For this review, take the finished solid that the model builds, in its own axes (mm). Face numbers are marked on the shaded views. A direction names the side the tool comes from. Coordinates: 2 decimals unless noted, no trailing zeros. Write each loop counter-clockwise with the first axis right and the second up, starting at its lowest first coordinate (ties: lowest second). Pieces come first, ordered by that corner, then holes.
1) We need section D-D on y = -19. Write out the cut boundary in (x, z), then the cut area to 3 significant figures.
2) To check wall thickness, follow line 1 along X through (y, z) = (-15, -13); line 2 along X through (y, z) = (-3, -7); line 3 along Z through (x, y) = (-25, -3). State the ranges of each line that lie inside material, in increasing order.
3) We need section C-C on z = -83.82. Write out the cut boundary in (x, y).
4) Mouldability with a two-part tool opening along X and no side actions: class the marked faces 5, 6 and 7 as pulls with the +X half, pulls with the -X half, needs draft (parallel to the pull), parting line crosses it, or undercut.
5) Insertion check: P1, Ø1.5, axis at x = -21.5, y = -73, coming from the +Z side; P2, Ø7.5, axis at x = -25.4, z = -7.62, coming from the +Y side; P3, Ø10, axis at x = -3, z = -16.5, coming from the -Y side; P4, Ø18, axis at x = -11, y = -12.5, coming from the -Z side. Each pin has a flat end and moves straight along its axis. Give the tip position at first contact, or say it passes through.
6) For the marked faces 1, 2, 3 and 4, list the 3-axis set-ups (+Z, -Z, +X, -X, +Y, -Y) from which the entire face can be reached by the end or side of a thin tool; tool diameter is ignored.
7) We need section B-B on z = -20.5. Write out the cut boundary in (x, y), then the cut area to 3 significant figures.
from build123d import *

# Parameters (mm, degrees)
F0_W          = 101.6
F0_H          = 50.8
F1_DEPTH      = 6.35
F2_W          = 101.6
F2_H          = 6.35
F3_DEPTH      = 152.4
F3_DEPTH_BACK = 3.175
F8_R          = 4.7625
F9_DEPTH      = 6.35
F10_DEPTH     = 6.35
F11_DEPTH     = 6.35
F12_D         = 9.525


with BuildPart() as f1:
    # F0 (on Front) → F1 (new body)
    with BuildSketch(Plane.XZ):
        Rectangle(F0_W, F0_H)
    extrude(amount=F1_DEPTH)

    # F2 (on face) → F3 (join, two sides)
    with BuildSketch(Plane.XZ.offset(6.35)) as f3_sk:
        with Locations((0, -28.575)):
            Rectangle(F2_W, F2_H)
    extrude(amount=F3_DEPTH)
    extrude(f3_sk.sketch, amount=-F3_DEPTH_BACK)

    # F8 (on offset) → F9 (join)
    with BuildSketch(Plane.XZ.offset(25.4)):
        with BuildLine():
            Line((-50.8, -31.75), (-13.0057051322, -91.7641320492))
            Line((-13.0057051322, -91.7641320492), (-12.7835835223, -92.1168423107))
            ThreePointArc((-12.7835835223, -92.1168423107), (0, -99.06), (12.7835835223, -92.1168423107))
            Line((12.7835835223, -92.1168423107), (13.0057051322, -91.7641320492))
            Line((13.0057051322, -91.7641320492), (50.8, -31.75))
            Line((50.8, -31.75), (-50.8, -31.75))
        make_face()
        with Locations((0, -83.82)):
            Circle(F8_R, mode=Mode.SUBTRACT)
    extrude(amount=F9_DEPTH)

    # F5 (on face) → F10 (join)
    with BuildSketch(Plane(origin=(-50.8, 0, 0), x_dir=(0, -1, 0), z_dir=(-1, 0, 0))):
        Polygon((82.55, -25.4), (6.35, 25.4), (6.35, -25.4), align=None)
    extrude(amount=-F10_DEPTH)

    # F4 (on face) → F11 (join)
    with BuildSketch(Plane.YZ.offset(50.8)):
        Polygon((-82.55, -25.4), (-6.35, -25.4), (-6.35, 25.4), align=None)
    extrude(amount=-F11_DEPTH)

    # F12 (through all)
    with Locations(Plane.XZ.offset(6.35)):
        with Locations((-25.4, -7.62)):
            Hole(F12_D / 2)


solid = f1.part
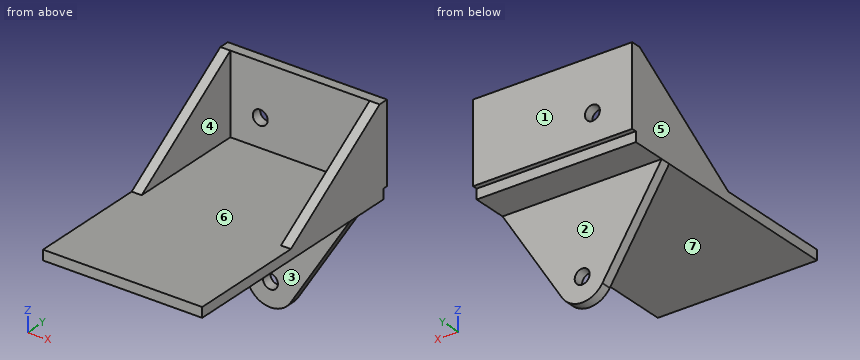
Result:
1. outline: (-50.8, -31.75) - (50.8, -31.75) - (50.8, 16.97) - (44.45, 16.97) - (44.45, -25.4) - (-44.45, -25.4) - (-44.45, 16.97) - (-50.8, 16.97) - close
1. area: 1,180 mm2
2. line 1: x = -50.8 to -44.45, 44.45 to 50.8
2. line 2: x = -50.8 to -30.12, -20.68 to 50.8
2. line 3: z = -25.4 to -12.37, -2.87 to 25.4
3. outline: (-18.01, -31.75) - (-4.76, -31.75) - (-4.76, -25.4) - (-18.01, -25.4) - close; (4.76, -31.75) - (18.01, -31.75) - (18.01, -25.4) - (4.76, -25.4) - close
4. face 5: pulls with the -X half
4. face 6: undercut
4. face 7: needs draft
5. P1: stops at z = -25.4
5. P2: passes through
5. P3: stops at y = -6.35
5. P4: stops at z = -31.75
6. face 1: +Z, -Z, +X, -X, +Y
6. face 2: -Z, +X, -X, +Y
6. face 3: -Z, +X, -X, -Y
6. face 4: +Z, -Y
7. outline: (-50.8, -75.2) - (-44.45, -75.2) - (-44.45, -6.35) - (44.45, -6.35) - (44.45, -75.2) - (50.8, -75.2) - (50.8, 0) - (-50.8, 0) - close
7. area: 1,520 mm2
